from build123d import *

# Parameters (mm, degrees)
F1_DEPTH = 1.8415
F2_W     = 1.016
F2_H     = 2.032
F3_DEPTH = 25.4


with BuildPart() as f1:
    # F0 (on Front) → F1 (new body, symmetric)
    with BuildSketch(Plane.XZ):
        Polygon((0, 0), (0, -15.875), (0.3048, -15.875), (0.3048, 0), (0.3048, 0.3048), (-1.131116, 0.3048), (-4.489804, 9.532717), (-7.403488, 11.460087), (-7.569124, 11.199027), (-4.777688, 9.427936), (-1.3462, 0), align=None)
    extrude(amount=F1_DEPTH, both=True)

    # F2 (on face) → F3 (cut)
    with BuildSketch(Plane(origin=(0, 0, 0), x_dir=(0, -1, 0), z_dir=(-1, 0, 0))):
        with Locations((-1.3335, -1.016)):
            Rectangle(F2_W, F2_H)
    extrude(amount=-F3_DEPTH, mode=Mode.SUBTRACT)


solid = f1.part
Check sheet for the modelled part. Datum: model origin and axes. Units: mm. A direction names the side the tool comes from. Round coordinates to 2 decimals unless told otherwise and drop trailing zeros. Order: outer loops, then holes, each group sorted by start corner. A loop starts at its lowest first (then second) coordinate and runs counter-clockwise, first axis right, second up.
Q1. Cross-section at A-A, the plane y = 1.1. Enter the section's corners in (x, z) (3 decimals).
Filled sheet:
outline: (-7.569, 11.199) - (-4.778, 9.428) - (-1.346, 0) - (0.305, 0) - (0.305, 0.305) - (-1.131, 0.305) - (-4.49, 9.533) - (-7.403, 11.46) - close; (0, -15.875) - (0.305, -15.875) - (0.305, -2.032) - (0, -2.032) - close
Q2. Scan lines: L1, parallel to X at y = -0.4, z = -8; L2, parallel to Z at x = -5.75, y = -1.35. Record each from-to range of solid material in increasing order.
Filled sheet:
L1: x = 0 to 0.3
L2: z = 10.04 to 10.37
Q3. Cross-section at B-B, the plane z = -4.25. Enter the section's corners in (x, y).
Filled sheet:
outline: (0, -1.84) - (0.3, -1.84) - (0.3, 1.84) - (0, 1.84) - close
Q4. Set-up check for faces 4 (the face through (0.305, 0, -8)), 5 (the face through (0, 0, 0.305)), 6 (the face through (0, 0, -8)): record each of +Z, -Z, +X, -X, +Y, -Y from which the full face is reachable in a straight line by a thin tool's end or side.
Filled sheet:
face 4: +Z, -Z, +X, +Y, -Y
face 5: +Z, +X, +Y, -Y
face 6: -Z, -X, +Y, -Y
Q5. Cross-section at C-C, the plane x = -2.25. Enter the section's corners in (y, z), plus the area to 3 significant figures.
Filled sheet:
outline: (-1.84, 2.48) - (1.84, 2.48) - (1.84, 3.38) - (-1.84, 3.38) - close
area: 3.30 mm2
Q6. Draft check along Z on faces 1 (the face through (-6.193, -0.026, 10.326)), 2 (the face through (-3, 1.842, 5)), 3 (the face through (-2.787, -0.026, 4.854)). Enter one of: pulls with the +Z half, pulls with the -Z half, needs draft (parallel to the pull), parting line crosses it, or undercut.
Filled sheet:
face 1: pulls with the -Z half
face 2: needs draft
face 3: pulls with the +Z half
Q7. Depth check by flat-ended pin: P1, Ø0.7, axis at x = -0.5, y = -0.5, coming from the +Z side; P2, Ø1.5, axis at x = -6.5, y = 1.5, coming from the +Z side; P3, Ø1, axis at x = -3, z = 2, coming from the -Y side. Enter the tip coordinate at first touch or a pass-through.
Filled sheet:
P1: stops at z = 0.3
P2: stops at z = 11.36
P3: passes through
